Work out the finished part from the listing and answer in its coordinate system (mm). Face numbers are marked on the shaded views. Give positions to 0.01 mm unless a question says otherwise; leave off trailing zeros. Order: outer loops, then holes, each group sorted by start corner. A loop starts at its lowest first (then second) coordinate and runs counter-clockwise, first axis right, second up. Notation, with made-up numbers: (80.25, 6.5) - (88.25, 6.5) arc R5 cw to (88.25, 15.5) - close; hole circle Ø11 at (55.25, -14). An arc over 180 degrees is marked (long way). Put each result on its own line as item: value.
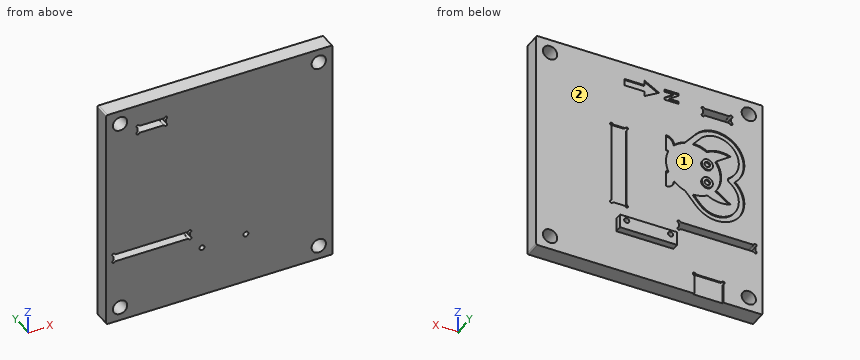
```python
from build123d import *

# Parameters (mm, degrees)
SKICA1_W                        = 164
SKICA1_H                        = 164
P_IDAT_VYSUNUT_M1_DEPTH         = 12
SKICA2_R                        = 5.2
ODEBRAT_VYSUNUT_M1_DEPTH        = 117.584733134
SKICA3_W                        = 55.4
SKICA3_H                        = 5.4
SKICA3_W_2                      = 20.4
ODEBRAT_VYSUNUT_M2_DEPTH        = 117.584733134
ODEBRAT_VYSUNUT_M3_DEPTH        = 1
ZAOBLIT1_R                      = 1
SKICA10_W                       = 41.4
SKICA10_H                       = 10
P_IDAT_VYSUNUT_M2_DEPTH         = 5
ODEBRAT_VYSUNUT_M6_DEPTH        = 117.584733134
ODEBRAT_VYSUNUT_M6_DEPTH_BACK   = 117.584733134
SKICA10_3_R                     = 1.85
SKICA11_W                       = 21
SKICA11_H                       = 15.5
SKICA11_W_2                     = 11
SKICA11_H_2                     = 61
ODEBRAT_VYSUNUT_M7_DEPTH        = 1
SKICA12_R                       = 1
ODEBRAT_VYSUNUT_M8_DEPTH        = 117.584733134
ZAOBLIT2_R                      = 1
SKICA13_R                       = 1
ODEBRAT_VYSUNUT_M9_DEPTH        = 1
ZAOBLIT3_R                      = 1
ODEBRAT_START                   = 11
ODEBRAT_VYSUNUT_M11_OUTLINE_R   = 4
ODEBRAT_VYSUNUT_M11_OUTLINE_R_2 = 2
ODEBRAT_VYSUNUT_M11_DEPTH       = 1


# Read off the part's stored shape, not the designer's step: Odebrat vysunutím11
with BuildPart() as part:
    # Skica1 → Přidat vysunutím1 (new body)
    with BuildSketch(Plane(origin=(0, 0, 0), x_dir=(1, 0, 0), z_dir=(0, 1, 0))):
        Rectangle(SKICA1_W, SKICA1_H)
    extrude(amount=P_IDAT_VYSUNUT_M1_DEPTH)

    # Skica2 → Odebrat vysunutím1 (cut, through all)
    with BuildSketch(Plane(origin=(0, 12, 0), x_dir=(1, 0, 0), z_dir=(0, 1, 0))):
        with Locations(Location((-72, 72, 0), (0, 0, 270))):
            Circle(SKICA2_R)
        with Locations(Location((72, 72, 0), (0, 0, 270))):
            Circle(SKICA2_R)
        with Locations(Location((-72, -72, 0), (0, 0, 270))):
            Circle(SKICA2_R)
        with Locations(Location((72, -72, 0), (0, 0, 270))):
            Circle(SKICA2_R)
    extrude(amount=-ODEBRAT_VYSUNUT_M1_DEPTH, mode=Mode.SUBTRACT)

    # Skica3 → Odebrat vysunutím2 (cut, through all)
    with BuildSketch(Plane(origin=(0, 12, 0), x_dir=(1, 0, 0), z_dir=(0, 1, 0))):
        with Locations((-49, 32)):
            Rectangle(SKICA3_W, SKICA3_H)
        with Locations((-49, -63)):
            Rectangle(SKICA3_W_2, SKICA3_H)
    extrude(amount=-ODEBRAT_VYSUNUT_M2_DEPTH, mode=Mode.SUBTRACT)

    # Skica4 → Odebrat vysunutím3 (cut)
    with BuildSketch(Plane(origin=(0, 12, 0), x_dir=(1, 0, 0), z_dir=(0, 1, 0))):
        Polygon((3.392304845, -61), (-7, -67), (3.392304845, -73), (3.392304845, -69.5), (18, -69.5), (18, -64.5), (3.392304845, -64.5), align=None)
        Polygon((-11, -63.025641026), (-11, -64.642227564), (-17.580528846, -69.179487179), (-11, -69.179487179), (-11, -70.974358974), (-21, -70.974358974), (-21, -69.345753205), (-14.439503205, -64.820512821), (-21, -64.820512821), (-21, -63.025641026), align=None)
    extrude(amount=-ODEBRAT_VYSUNUT_M3_DEPTH, mode=Mode.SUBTRACT)

    # Zaoblit1
    zaoblit1_edges = [part.edges().sort_by_distance(p)[0] for p in [
        (82, 6, 82),
        (-82, 6, 82),
        (-82, 6, -82),
        (82, 6, -82),
    ]]
    fillet(zaoblit1_edges, radius=ZAOBLIT1_R)

    # Skica10 → Přidat vysunutím2 (add)
    with BuildSketch(Plane(origin=(0, 12, 0), x_dir=(1, 0, 0), z_dir=(0, 1, 0))):
        with Locations((3.25, 47)):
            Rectangle(SKICA10_W, SKICA10_H)
    extrude(amount=P_IDAT_VYSUNUT_M2_DEPTH)

    # Skica10<3> → Odebrat vysunutím6 (cut, two sides: drawn at the far end of the back side and taken through both)
    with BuildSketch(Plane(origin=(0, 12, 0), x_dir=(1, 0, 0), z_dir=(0, 1, 0)).offset(-ODEBRAT_VYSUNUT_M6_DEPTH_BACK)):
        with Locations(Location((-12.625, 45.13, 0), (0, 0, 270))):
            Circle(SKICA10_3_R)
        with Locations(Location((19.125, 45.13, 0), (0, 0, 270))):
            Circle(SKICA10_3_R)
    extrude(amount=ODEBRAT_VYSUNUT_M6_DEPTH + ODEBRAT_VYSUNUT_M6_DEPTH_BACK, mode=Mode.SUBTRACT)

    # Skica11 → Odebrat vysunutím7 (cut)
    with BuildSketch(Plane(origin=(0, 12, 0), x_dir=(1, 0, 0), z_dir=(0, 1, 0))):
        with Locations((-43, 74.25)):
            Rectangle(SKICA11_W, SKICA11_H)
        with Locations((22, -0.5)):
            Rectangle(SKICA11_W_2, SKICA11_H_2)
    extrude(amount=-ODEBRAT_VYSUNUT_M7_DEPTH, mode=Mode.SUBTRACT)

    # Skica12 → Odebrat vysunutím8 (cut, through all)
    with BuildSketch(Plane(origin=(0, 12, 0), x_dir=(1, 0, 0), z_dir=(0, 1, 0))):
        with Locations((-76.7, 34.7)):
            Circle(SKICA12_R)
        with Locations((-76.7, 29.3)):
            Circle(SKICA12_R)
        with Locations((-21.3, 29.3)):
            Circle(SKICA12_R)
        with Locations((-21.3, 34.7)):
            Circle(SKICA12_R)
        with Locations((-59.2, -60.3)):
            Circle(SKICA12_R)
        with Locations((-59.2, -65.7)):
            Circle(SKICA12_R)
        with Locations((-38.8, -65.7)):
            Circle(SKICA12_R)
        with Locations((-38.8, -60.3)):
            Circle(SKICA12_R)
    extrude(amount=-ODEBRAT_VYSUNUT_M8_DEPTH, mode=Mode.SUBTRACT)

    # Zaoblit2
    zaoblit2_edges = [part.edges().sort_by_distance(p)[0] for p in [
        (-75.7, 6, -34.7),
        (-22.3, 6, -34.7),
        (-76.7, 6, -30.3),
        (-22.3, 6, -29.3),
        (-39.8, 6, 60.3),
        (-58.2, 6, 60.3),
        (-59.2, 6, 64.7),
        (-39.8, 6, 65.7),
        (-59.2, 6, 61.3),
        (-21.3, 6, -33.7),
        (-21.3, 6, -30.3),
        (-75.7, 6, -29.3),
        (-58.2, 6, 65.7),
        (-38.8, 6, 64.7),
        (-38.8, 6, 61.3),
        (-76.7, 6, -33.7),
    ]]
    fillet(zaoblit2_edges, radius=ZAOBLIT2_R)

    # Skica13 → Odebrat vysunutím9 (cut)
    with BuildSketch(Plane(origin=(0, 12, 0), x_dir=(1, 0, 0), z_dir=(0, 1, 0))):
        with Locations((-53.5, 66.5)):
            Circle(SKICA13_R)
        with Locations((-32.5, 66.5)):
            Circle(SKICA13_R)
        with Locations((16.5, 30)):
            Circle(SKICA13_R)
        with Locations((27.5, 30)):
            Circle(SKICA13_R)
        with Locations((16.5, -31)):
            Circle(SKICA13_R)
        with Locations((27.5, -31)):
            Circle(SKICA13_R)
    extrude(amount=-ODEBRAT_VYSUNUT_M9_DEPTH, mode=Mode.SUBTRACT)

    # Zaoblit3
    zaoblit3_edges = [part.edges().sort_by_distance(p)[0] for p in [
        (-53.5, 11.5, -67.5),
        (-52.5, 11.5, -66.5),
        (27.5, 11.5, 30),
        (26.5, 11.5, 31),
        (-32.5, 11.5, -67.5),
        (-33.5, 11.5, -66.5),
        (16.5, 11.5, -29),
        (17.5, 11.5, -30),
        (26.5, 11.5, -30),
        (27.5, 11.5, -29),
        (16.5, 11.5, 30),
        (17.5, 11.5, 31),
    ]]
    fillet(zaoblit3_edges, radius=ZAOBLIT3_R)

    # Odebrat vysunutím11 outline → Odebrat vysunutím11 (cut)
    # profile 1 of 3: a face of its own
    with BuildSketch(Plane(origin=(0, 0, 0), x_dir=(1, 0, 0), z_dir=(0, 1, 0)).offset(ODEBRAT_START)):
        with BuildLine():
            ThreePointArc((-25.86889032, -34.537055815), (-21.651463985, -32.614549434), (-17.989824292, -29.772875555))
            ThreePointArc((-17.989824292, -29.772875555), (-16.143608013, -33.837823652), (-12, -35.5))
            Line((-12, -35.5), (-12, -23.508301528))
            ThreePointArc((-12, -23.508301528), (-12.908552323, -23.577537842), (-13.796121859, -23.783647786))
            ThreePointArc((-13.796121859, -23.783647786), (-12, -15.5), (-13.796121859, -7.216352214))
            ThreePointArc((-13.796121859, -7.216352214), (-12.908552323, -7.422462158), (-12, -7.491698472))
            Line((-12, -7.491698472), (-12, 4.5))
            ThreePointArc((-12, 4.5), (-16.143608013, 2.837823652), (-17.989824292, -1.227124445))
            ThreePointArc((-17.989824292, -1.227124445), (-21.651463985, 1.614549434), (-25.86889032, 3.537055815))
            Line((-25.86889032, 3.537055815), (-33.674320761, 12.533542588))
            ThreePointArc((-33.674320761, 12.533542588), (-62.826546549, 13.664932048), (-62.092346854, -15.5))
            ThreePointArc((-62.092346854, -15.5), (-62.826546549, -44.664932048), (-33.674320761, -43.533542588))
            Line((-33.674320761, -43.533542588), (-25.86889032, -34.537055815))
        make_face()
        with Locations((-42, -22.502075382)):
            Circle(ODEBRAT_VYSUNUT_M11_OUTLINE_R, mode=Mode.SUBTRACT)
        with BuildLine():
            ThreePointArc((-57.722697741, -17.158534068), (-56.840402867, -15.5), (-57.722697741, -13.841465932))
            ThreePointArc((-57.722697741, -13.841465932), (-60.761452982, 10.031999011), (-36.695667957, 9.912195392))
            Line((-36.695667957, 9.912195392), (-32, 4.5))
            ThreePointArc((-32, 4.5), (-37.176380902, 3.818516526), (-42, 1.820508076))
            ThreePointArc((-42, 1.820508076), (-50.256885145, 4.423893962), (-58.840402867, 3.293852416))
            Line((-58.840402867, 3.293852416), (-48.383040886, -4.028471273))
            ThreePointArc((-48.383040886, -4.028471273), (-52, -15.5), (-48.383040886, -26.971528727))
            Line((-48.383040886, -26.971528727), (-58.840402867, -34.293852416))
            ThreePointArc((-58.840402867, -34.293852416), (-50.256885145, -35.423893962), (-42, -32.820508076))
            ThreePointArc((-42, -32.820508076), (-37.176380902, -34.818516526), (-32, -35.5))
            Line((-32, -35.5), (-36.695667957, -40.912195392))
            ThreePointArc((-36.695667957, -40.912195392), (-60.761452982, -41.031999011), (-57.722697741, -17.158534068))
        make_face(mode=Mode.SUBTRACT)
        with Locations((-42, -8.497924618)):
            Circle(ODEBRAT_VYSUNUT_M11_OUTLINE_R, mode=Mode.SUBTRACT)
    # profile 2 of 3: a face of its own
    with BuildSketch(Plane(origin=(0, 0, 0), x_dir=(1, 0, 0), z_dir=(0, 1, 0)).offset(ODEBRAT_START)):
        with Locations((-42, -22.502075382)):
            Circle(ODEBRAT_VYSUNUT_M11_OUTLINE_R_2)
    # profile 3 of 3: a face of its own
    with BuildSketch(Plane(origin=(0, 0, 0), x_dir=(1, 0, 0), z_dir=(0, 1, 0)).offset(ODEBRAT_START)):
        with Locations((-42, -8.497924618)):
            Circle(ODEBRAT_VYSUNUT_M11_OUTLINE_R_2)
    extrude(amount=ODEBRAT_VYSUNUT_M11_DEPTH, mode=Mode.SUBTRACT)


solid = part.part
```
(1) Straight lines are drawn through the part: line 1 (Z direction, x = -41, y = 3.25); line 2 (X direction, y = 5, z = -29); line 3 (X direction, y = 1, z = -46.5). For each, find the intervals that lie inside material, in ascending order.
Geometry check:
line 1: z = -82 to -34.7, -29.3 to 60.3, 65.7 to 82
line 2: x = -82 to -77.65, -75.68 to -22.32, -20.35 to 82
line 3: x = -82 to -13.87, -11.38 to 17.88, 20.37 to 82
(2) Section C-C, the plane z = -55.5 is taken. Write down the section's boundary in (x, y).
Geometry check:
outline: (-82, 0) - (82, 0) - (82, 12) - (-82, 12) - close
(3) Given pin 1 (2.5 mm diameter, centred on x = -42, z = 8.5, fed in from +Y); pin 2 (6.5 mm diameter, centred on x = -17, z = 67.5, fed in from +Y), each flat-ended and moving along its own axis, determine where each tip first touches the part or whether it passes through.
Geometry check:
pin 1: stops at y = 11
pin 2: stops at y = 12
(4) Determine the mould class of the marked faces 1 and 2 for opening direction Z: pulls with the +Z half, pulls with the -Z half, needs draft (parallel to the pull), parting line crosses it, or undercut.
Geometry check:
face 1: undercut
face 2: needs draft
(5) Section B-B, the plane y = 4.5 is taken. Count the separate pieces of the cut face and the enclosed holes in it, then the cut area to 3 significant figures.
Geometry check:
separate pieces: 1
enclosed holes: 8
area: 26,100 mm²
(6) Section A-A, the plane x = 35.5 is taken. Write down the section's boundary in (y, z), then the cut area to 3 significant figures.
Geometry check:
outline: (0, -82) - (12, -82) - (12, 82) - (0, 82) - close
area: 1,970 mm²
